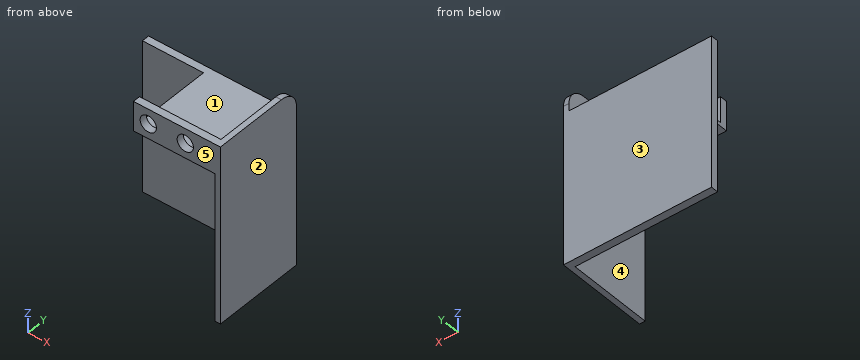
```python
from build123d import *

# Parameters (mm, degrees)
BOSS_EXTRUDE1_DEPTH = 22
SKETCH4_W           = 48
SKETCH4_H           = 25
BOSS_EXTRUDE3_DEPTH = 1.5
SKETCH5_W           = 40
SKETCH5_H           = 41
BOSS_EXTRUDE4_DEPTH = 2
CUT_EXTRUDE2_REACH  = 54.7
SKETCH6_R           = 2.2
LPATTERN2_COUNT     = 2
LPATTERN2_PITCH     = 10
FILLET2_R           = 5


with BuildPart() as part:
    # Sketch1 → Boss-Extrude1 (new body)
    with BuildSketch(Plane(origin=(0, 0, 0), x_dir=(0, 0, -1), z_dir=(1, 0, 0))):
        Polygon((-8, -25), (0, -25), (0, 0), (-1, 0), (-1, -23), (-8, -23), align=None)
    extrude(amount=BOSS_EXTRUDE1_DEPTH)

    # Sketch4 → Boss-Extrude3 (add)
    with BuildSketch(Plane(origin=(22, 0, 0), x_dir=(0, 0, -1), z_dir=(1, 0, 0))):
        with Locations((16, -12.5)):
            Rectangle(SKETCH4_W, SKETCH4_H)
    extrude(amount=BOSS_EXTRUDE3_DEPTH)

    # Sketch5 → Boss-Extrude4 (add)
    with BuildSketch(Plane(origin=(0, 0, 0), x_dir=(1, 0, 0), z_dir=(0, 1, 0))):
        with Locations((3.5, 19.5)):
            Rectangle(SKETCH5_W, SKETCH5_H)
    extrude(amount=-BOSS_EXTRUDE4_DEPTH)

    # Sketch6 → Cut-Extrude2 (cut, up to next)
    with BuildSketch(Plane.XZ.offset(25), mode=Mode.PRIVATE) as cut_extrude2_sk1:
        with Locations(Location((14, 4, 0), (0, 0, 270))):
            Circle(SKETCH6_R)
    cut_extrude2_tool1 = extrude(cut_extrude2_sk1.sketch, amount=-CUT_EXTRUDE2_REACH, mode=Mode.PRIVATE) & part.part
    cut_extrude2 = cut_extrude2_tool1.solids().sort_by_distance((14, -25, 4))[0]
    add(cut_extrude2, mode=Mode.SUBTRACT)

    # LPattern2: Cut-Extrude2 ×2
    with Locations(*[(-i * LPATTERN2_PITCH, 0, 0) for i in range(1, LPATTERN2_COUNT)]):
        add(cut_extrude2, mode=Mode.SUBTRACT)

    # Fillet2
    fillet2_edges = [part.edges().sort_by_distance(p)[0] for p in [
        (22.75, 0, 8),
    ]]
    fillet(fillet2_edges, radius=FILLET2_R)


solid = part.part
```
Work out the finished part from the listing and answer in its coordinate system (mm). Face numbers are marked on the shaded views. A direction names the side the tool comes from. Coordinates: 2 decimals unless noted, no trailing zeros. Write each loop counter-clockwise with the first axis right and the second up, starting at its lowest first coordinate (ties: lowest second). Pieces come first, ordered by that corner, then holes. Notation, with made-up numbers: (58.25, -12) - (91.25, -12) arc R23 ccw to (91.25, 25) - close; hole circle Ø6 at (43, 85.25). An arc over 180 degrees is marked (long way). Answer as a JSON object with one key per item and string values.
Q1. Which of the six approach directions +Z, -Z, +X, -X, +Y, -Y give full straight-line access (tool end or side, diameter ignored) to the marked faces 1 and 2?
Results list:
{"face 1": "+Z, -X, +Y", "face 2": "+Z, -Z, +X, +Y, -Y"}
Q2. Find section D-D (x = 7). Write down the section's boundary in (y, z).
Results list:
{"outline": "(-25, 0) - (-2, 0) - (-2, -40) - (0, -40) - (0, 1) - (-23, 1) - (-23, 8) - (-25, 8) - close"}
Q3. Find section A-A (x = 14). Write down the section's boundary in (y, z), plus the area to 3 significant figures.
Results list:
{"outline": "(-25, 0) - (-2, 0) - (-2, -40) - (0, -40) - (0, 1) - (-23, 1) - (-23, 1.8) - (-25, 1.8) - close; (-25, 6.2) - (-23, 6.2) - (-23, 8) - (-25, 8) - close", "area": "110 mm^2"}
Q4. Find section B-B (z = 4). Write down the section's boundary in (x, y), plus the area to 3 significant figures.
Results list:
{"outline": "(0, -25) - (1.8, -25) - (1.8, -23) - (0, -23) - close; (6.2, -25) - (11.8, -25) - (11.8, -23) - (6.2, -23) - close; (16.2, -25) - (23.5, -25) - (23.5, -0.1) - (22, -0.1) - (22, -23) - (16.2, -23) - close", "area": "63.7 mm^2"}
Q5. For a pull along Y with two mould halves and no side action, classify the marked faces 3, 4 and 5 as pulls with the +Y half, pulls with the -Y half, needs draft (parallel to the pull), parting line crosses it, or undercut.
Results list:
{"face 3": "pulls with the +Y half", "face 4": "needs draft", "face 5": "pulls with the -Y half"}
Q6. Given pin 1 Ø2.5 at (x, z) = (14, 4) entering from +Y; pin 2 Ø6.5 at (x, y) = (14.5, -17) entering from -Z; pin 3 Ø4 at (x, z) = (18.5, -28) entering from -Y; pin 4 Ø3.5 at (x, z) = (5.5, 5.5) entering from +Y, each flat-ended and moving along its own axis, determine where each tip first touches the part or whether it passes through.
Results list:
{"pin 1": "passes through", "pin 2": "stops at z = 0", "pin 3": "stops at y = -2", "pin 4": "stops at y = -23"}
Q7. Consider L1, parallel to X at y = -23.75, z = 4; L2, parallel to X at y = -11.25, z = -13; L3, parallel to Z at x = 2, y = -14. Determine where each line is inside the solid, lowest interval first. Write a range as from..to.
Results list:
{"L1": "x = 0..1.8, 6.2..11.8, 16.2..23.5", "L2": "x = 22..23.5", "L3": "z = 0..1"}
Q8. Find section C-C (y = -12.25). Write down the section's boundary in (x, z), plus the area to 3 significant figures.
Results list:
{"outline": "(0, 0) - (22, 0) - (22, -40) - (23.5, -40) - (23.5, 8) - (22, 8) - (22, 1) - (0, 1) - close", "area": "94.0 mm^2"}
